The listing builds one solid part. Answer for the finished solid, in the listing's coordinates (mm). Face numbers are marked on the shaded views. A direction names the side the tool comes from. Round coordinates to 2 decimals unless told otherwise and drop trailing zeros. Write each loop counter-clockwise with the first axis right and the second up, starting at its lowest first coordinate (ties: lowest second). Pieces come first, ordered by that corner, then holes.
from build123d import *

# Parameters (mm, degrees)
CYLINDER022_R                        = 1.95
CYLINDER022_DEPTH                    = 10
CYLINDER021_R                        = 1.95
CYLINDER021_DEPTH                    = 10
BOX026_W                             = 2
BOX026_H                             = 6
BOX026_DEPTH                         = 5.9
BOX027_W                             = 2
BOX027_H                             = 6
BOX027_DEPTH                         = 5.9
CHAMFER004013007011015006009004_SIZE = 1
CYLINDER018_R                        = 2.525
CYLINDER018_DEPTH                    = 37
CYLINDER019_R                        = 4.75
CYLINDER019_DEPTH                    = 8
CYLINDER017_R                        = 2.65
CYLINDER017_DEPTH                    = 2
CYLINDER016_R                        = 6.55
CYLINDER016_DEPTH                    = 5
BOX030_W                             = 12
BOX030_H                             = 8
BOX030_DEPTH                         = 10
BOX024_W                             = 31
BOX024_H                             = 20
BOX024_DEPTH                         = 25
CHAMFER004013007011015006009005_SIZE = 17
CHAMFER004013007011015006009006_SIZE = 1
BOX028_W                             = 6
BOX028_H                             = 7
BOX028_DEPTH                         = 1
BOX029_W                             = 6
BOX029_H                             = 7
BOX029_DEPTH                         = 1
CYLINDER020_R                        = 2.525
CYLINDER020_DEPTH                    = 10
BOX025_W                             = 20
BOX025_H                             = 20
BOX025_DEPTH                         = 5
FILLET001_R                          = 3
CHAMFER004013007011015006009007_SIZE = 0.4


with BuildPart() as cylinder022:
    # Cylinder022 → Cylinder022 (new body)
    with BuildSketch(Plane(origin=(24, 14, 41), x_dir=(1, 0, 0), z_dir=(0, -1, 0))):
        Circle(CYLINDER022_R)
    extrude(amount=CYLINDER022_DEPTH)


with BuildPart() as fusion004031:
    # Cylinder021 → Cylinder021 (new body)
    with BuildSketch(Plane(origin=(24, -4, 41), x_dir=(1, 0, 0), z_dir=(0, -1, 0))):
        Circle(CYLINDER021_R)
    extrude(amount=CYLINDER021_DEPTH)

    # Fusion004031: union Cylinder022
    add(cylinder022.part)


with BuildPart() as fusion004031_1:
    # Fusion004031 placement: moved
    add(fusion004031.part.moved(Location((1, 0, 0))))


with BuildPart() as cube026:
    # Box026 → Box026 (new body)
    with BuildSketch(Plane(origin=(46, -10, 47), x_dir=(1, 0, 0), z_dir=(0, 0, 1))):
        with Locations((1, 3)):
            Rectangle(BOX026_W, BOX026_H)
    extrude(amount=BOX026_DEPTH)


with BuildPart() as chamfer004013007011015006009004:
    # Box027 → Box027 (new body)
    with BuildSketch(Plane(origin=(46, 4, 47), x_dir=(1, 0, 0), z_dir=(0, 0, 1))):
        with Locations((1, 3)):
            Rectangle(BOX027_W, BOX027_H)
    extrude(amount=BOX027_DEPTH)

    # Fusion004032: union Cube026
    add(cube026.part)


with BuildPart() as chamfer004013007011015006009004_1:
    # Fusion004032 placement: moved
    add(chamfer004013007011015006009004.part.moved(Location((0, 0, -5.1))))

    # Chamfer004013007011015006009004
    chamfer004013007011015006009004_edges = [chamfer004013007011015006009004_1.edges().sort_by_distance(p)[0] for p in [
        (48, 7, 47.8),
        (48, -7, 47.8),
    ]]
    chamfer(chamfer004013007011015006009004_edges, length=CHAMFER004013007011015006009004_SIZE)


with BuildPart() as chamfer004013007011015006009004_2:
    # Chamfer004013007011015006009004 placement: moved
    add(chamfer004013007011015006009004_1.part.moved(Location((0, 0, 0.1))))


with BuildPart() as cylinder018:
    # Cylinder018 → Cylinder018 (new body)
    with BuildSketch(Plane(origin=(14, 0, 45), x_dir=(0, 0, -1), z_dir=(1, 0, 0))):
        Circle(CYLINDER018_R)
    extrude(amount=CYLINDER018_DEPTH)


with BuildPart() as fusion004035:
    # Cylinder019 → Cylinder019 (new body)
    with BuildSketch(Plane(origin=(14, 0, 45), x_dir=(0, 0, -1), z_dir=(1, 0, 0))):
        Circle(CYLINDER019_R)
    extrude(amount=CYLINDER019_DEPTH)

    # Fusion004035: union Cylinder018
    add(cylinder018.part)


with BuildPart() as cylinder017:
    # Cylinder017 → Cylinder017 (new body)
    with BuildSketch(Plane.XY.offset(3)):
        Circle(CYLINDER017_R)
    extrude(amount=CYLINDER017_DEPTH)


with BuildPart() as cut028006004005015:
    # Cylinder016 → Cylinder016 (new body)
    with BuildSketch(Plane.XY):
        Circle(CYLINDER016_R)
    extrude(amount=CYLINDER016_DEPTH)

    # Cut028006004005015: cut Cylinder017
    add(cylinder017.part, mode=Mode.SUBTRACT)


with BuildPart() as cut028006004005015_1:
    # Cut028006004005015 placement: moved
    add(cut028006004005015.part.moved(Location((22, 0, 33))))


with BuildPart() as fusion004030:
    # Box030 → Box030 (new body)
    with BuildSketch(Plane(origin=(7, -4, 28), x_dir=(1, 0, 0), z_dir=(0, 0, 1))):
        with Locations((6, 4)):
            Rectangle(BOX030_W, BOX030_H)
    extrude(amount=BOX030_DEPTH)

    # Fusion004030: union Cut028006004005015
    add(cut028006004005015_1.part)


with BuildPart() as cut028006004005011003:
    # Box024 → Box024 (new body)
    with BuildSketch(Plane(origin=(16, -10, 35), x_dir=(1, 0, 0), z_dir=(0, 0, 1))):
        with Locations((15.5, 10)):
            Rectangle(BOX024_W, BOX024_H)
    extrude(amount=BOX024_DEPTH)

    # Cut028006004005017: cut Fusion004030
    add(fusion004030.part, mode=Mode.SUBTRACT)

    # Chamfer004013007011015006009005
    chamfer004013007011015006009005_edges = [cut028006004005011003.edges().sort_by_distance(p)[0] for p in [
        (16, 0, 60),
    ]]
    chamfer(chamfer004013007011015006009005_edges, length=CHAMFER004013007011015006009005_SIZE)

    # Cut028006004005018: cut Fusion004035
    add(fusion004035.part, mode=Mode.SUBTRACT)

    # Chamfer004013007011015006009006
    chamfer004013007011015006009006_edges = [cut028006004005011003.edges().sort_by_distance(p)[0] for p in [
        (16, 7, 35),
        (16, -7, 35),
    ]]
    chamfer(chamfer004013007011015006009006_edges, length=CHAMFER004013007011015006009006_SIZE)

    # Fusion004025007: union Chamfer004013007011015006009004
    add(chamfer004013007011015006009004_2.part)

    # Cut028006004005011003: cut Fusion004031
    add(fusion004031_1.part, mode=Mode.SUBTRACT)


with BuildPart() as cube028:
    # Box028 → Box028 (new body)
    with BuildSketch(Plane(origin=(54, -10, 40), x_dir=(1, 0, 0), z_dir=(0, 0, 1))):
        with Locations((3, 3.5)):
            Rectangle(BOX028_W, BOX028_H)
    extrude(amount=BOX028_DEPTH)


with BuildPart() as cube029:
    # Box029 → Box029 (new body)
    with BuildSketch(Plane(origin=(54, 3, 40), x_dir=(1, 0, 0), z_dir=(0, 0, 1))):
        with Locations((3, 3.5)):
            Rectangle(BOX029_W, BOX029_H)
    extrude(amount=BOX029_DEPTH)


with BuildPart() as cylinder020:
    # Cylinder020 → Cylinder020 (new body)
    with BuildSketch(Plane(origin=(57, 0, 32), x_dir=(1, 0, 0), z_dir=(0, 0, 1))):
        Circle(CYLINDER020_R)
    extrude(amount=CYLINDER020_DEPTH)


with BuildPart() as bed_frame_mount_top:
    # Box025 → Box025 (new body)
    with BuildSketch(Plane(origin=(47, -10, 35), x_dir=(1, 0, 0), z_dir=(0, 0, 1))):
        with Locations((10, 10)):
            Rectangle(BOX025_W, BOX025_H)
    extrude(amount=BOX025_DEPTH)

    # Fillet001
    fillet001_edges = [bed_frame_mount_top.edges().sort_by_distance(p)[0] for p in [
        (67, -10, 37.5),
        (67, 10, 37.5),
    ]]
    fillet(fillet001_edges, radius=FILLET001_R)

    # Cut028006004005016: cut Cylinder020
    add(cylinder020.part, mode=Mode.SUBTRACT)


with BuildPart() as bed_frame_mount_top_1:
    # Cut028006004005016 placement: moved
    add(bed_frame_mount_top.part.moved(Location((0, 0, 6))))

    # Fusion004034: union Cube028, Cube029
    add(cube028.part)
    add(cube029.part)


with BuildPart() as bed_frame_mount_top_2:
    # Fusion004034 placement: moved
    add(bed_frame_mount_top_1.part.moved(Location((0, 0, 14))))

    # Fusion004025008: union Cut028006004005011003
    add(cut028006004005011003.part)

    # Chamfer004013007011015006009007
    chamfer004013007011015006009007_edges = [bed_frame_mount_top_2.edges().sort_by_distance(p)[0] for p in [
        (67, 0, 60),
        (55.5, 10, 60),
        (66.12132, 9.12132, 60),
        (55.5, -10, 60),
        (66.12132, -9.12132, 60),
        (40, 10, 60),
        (40, -10, 60),
        (16.5, 10, 35.5),
        (16, 10, 39.5),
        (32, 10, 35),
        (24.5, 10, 51.5),
        (24.5, -10, 51.5),
        (16.5, -10, 35.5),
        (16, -10, 39.5),
        (32, -10, 35),
    ]]
    chamfer(chamfer004013007011015006009007_edges, length=CHAMFER004013007011015006009007_SIZE)


solid = bed_frame_mount_top_2.part
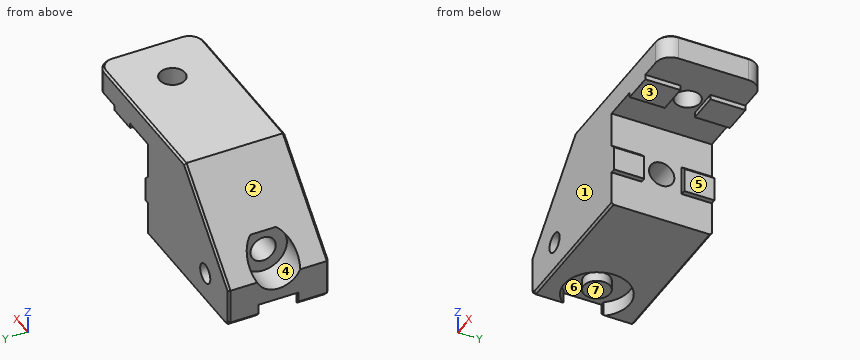
1. Given pin 1 (5.5 mm diameter, centred on y = 8, z = 45, fed in from +X); pin 2 (0.5 mm diameter, centred on x = 47.5, y = 8, fed in from -Z); pin 3 (0.5 mm diameter, centred on y = -5, z = 54.5, fed in from -X), each flat-ended and moving along its own axis, determine where each tip first touches the part or whether it passes through.
Geometry says:
pin 1: stops at x = 48
pin 2: stops at z = 42
pin 3: stops at x = 27.25
2. Section A-A on x = 57 is taken. Determine the outline of the cut face in (y, z) (3 decimals).
Geometry says:
outline: (-10, 54) - (-3, 54) - (-3, 55) - (-2.525, 55) - (-2.525, 60) - (-9.6, 60) - (-10, 59.6) - close; (2.525, 55) - (3, 55) - (3, 54) - (10, 54) - (10, 59.6) - (9.6, 60) - (2.525, 60) - close
3. Section D-D on x = 29.5 is taken. Determine the outline of the cut face in (y, z) (3 decimals), plus the area to 3 significant figures.
Geometry says:
outline: (-10, 35.4) - (-9.6, 35) - (9.6, 35) - (10, 35.4) - (10, 55.934) - (9.6, 56.5) - (-9.6, 56.5) - (-10, 55.934) - close; hole circle Ø5.05 at (0, 45)
area: 410 mm2
4. Section B-B on z = 37 is taken. Determine the outline of the cut face in (x, y).
Geometry says:
outline: (16, -9.6) - (16.4, -10) - (47, -10) - (47, 10) - (16.4, 10) - (16, 9.6) - (16, 4) - (16.81, 4) arc R6.55 cw (long way) to (16.81, -4) - (16, -4) - close; circle Ø5.3 at (22, 0)
5. For a pull along Z with two mould halves and no side action, classify the marked faces 1, 2, 3 and 4 as released by +Z, released by -Z, zero draft, split by the parting line, or undercut.
Geometry says:
face 1: zero draft
face 2: released by +Z
face 3: released by -Z
face 4: undercut
6. A tool of negligible diameter and unlimited length cuts with its end or side. For the marked faces 5, 6 and 7, from which of +Z, -Z, +X, -X, +Y, -Y can it reach the whole face along a straight path? Write none if from no direction.
Geometry says:
face 5: -Z, +X, +Y, -Y
face 6: -Z
face 7: -Z, -X
7. Section C-C on z = 39.75 is taken. Determine the outline of the cut face in (x, y), plus the area to 3 significant figures.
Geometry says:
outline: (16, -9.6) - (16.4, -10) - (23.5, -10) - (23.5, -4) - (26.5, -4) - (26.5, -10) - (47, -10) - (47, 10) - (26.5, 10) - (26.5, 4) - (23.5, 4) - (23.5, 10) - (16.4, 10) - (16, 9.6) - close
area: 584 mm2
8. Straight lines are drawn through the part: line 1 along Y through (x, z) = (22, 37); line 2 along X through (y, z) = (-8.35, 41); line 3 along Z through (x, y) = (60.5, -1.25). For each, find the intervals that lie inside material, in ascending order.
Geometry says:
line 1: y = -10 to -6.55, -2.65 to 2.65, 6.55 to 10
line 2: x = 16 to 23.05, 26.95 to 47
line 3: z = 55 to 60
